Verification items for the finished model (mm, model axes). A direction names the side the tool comes from. Round coordinates to 2 decimals unless told otherwise and drop trailing zeros. Order: outer loops, then holes, each group sorted by start corner. A loop starts at its lowest first (then second) coordinate and runs counter-clockwise, first axis right, second up. Notation, with made-up numbers: M 46,32 L 56,32 A21 ccw 56,41 Z; hole C 1.25,-22.5 d8. An arc over 180 degrees is marked long. Answer as a JSON object with one key per item and string values. Group by question number.
```python
from build123d import *

# Parameters (mm, degrees)
F1_DEPTH = 38.1
F2_R     = 15.875
F3_DEPTH = 31.75
F5_DEPTH = 31.75


with BuildPart() as f1:
    # F0 (on Top) → F1 (new body)
    with BuildSketch(Plane.XY):
        with BuildLine():
            Line((17.5179102392, -5.2510727335), (17.5179102392, 5.2510727335))
            ThreePointArc((17.5179102392, 5.2510727335), (17.276294132, 5.9983835377), (17.0028141207, 6.7346310944))
            ThreePointArc((17.0028141207, 6.7346310944), (-18.288, 0), (17.0028141207, -6.7346310944))
            ThreePointArc((17.0028141207, -6.7346310944), (17.276294132, -5.9983835377), (17.5179102392, -5.2510727335))
        make_face()
        with BuildLine():
            ThreePointArc((17.0028141207, 6.7346310944), (17.276294132, 5.9983835377), (17.5179102392, 5.2510727335))
            ThreePointArc((17.5179102392, 5.2510727335), (23.5952406288, 0), (17.5179102392, -5.2510727335))
            ThreePointArc((17.5179102392, -5.2510727335), (17.276294132, -5.9983835377), (17.0028141207, -6.7346310944))
            ThreePointArc((17.0028141207, -6.7346310944), (25.1441620986, 0), (17.0028141207, 6.7346310944))
        make_face()
    extrude(amount=-F1_DEPTH)

    # F2 (on face) → F3 (cut)
    with BuildSketch(Plane(origin=(0, 0, -38.1), x_dir=(1, 0, 0), z_dir=(0, 0, -1))):
        Circle(F2_R)
    extrude(amount=-F3_DEPTH, mode=Mode.SUBTRACT)

    # F4 (on face) → F5 (cut)
    with BuildSketch(Plane(origin=(0, 0, -38.1), x_dir=(1, 0, 0), z_dir=(0, 0, -1))):
        with BuildLine():
            ThreePointArc((17.0028141207, -6.7346310944), (25.1441620986, 0), (17.0028141207, 6.7346310944))
            Line((17.0028141207, 6.7346310944), (17.5179102392, 5.2510727335))
            ThreePointArc((17.5179102392, 5.2510727335), (23.5952406288, 0), (17.5179102392, -5.2510727335))
            Line((17.5179102392, -5.2510727335), (17.0028141207, -6.7346310944))
        make_face()
    extrude(amount=-F5_DEPTH, mode=Mode.SUBTRACT)


solid = f1.part
```
Q1. Gauge pin test, flat ends, axial feed: pin 1 Ø12 at (y, z) = (-5, -28) entering from -X; pin 2 Ø1.5 at (y, z) = (7, -29.5) entering from -X; pin 3 Ø3 at (y, z) = (13, -25.5) entering from -X. Record the tip position at first contact, or that the pin passes through.
Q2. Cross-section at C-C, the plane z = -20. Record the cut outline in (x, y) (3 decimals), then the cut area to 3 significant figures.
Q3. Tool access check on faces 1 (the face through (17.257, -6.003, -22.447)), 2 (the face through (-15, 6, -38.1)), 3 (the face through (0, 0, -6.35)). Record the directions out of +Z, -Z, +X, -X, +Y, -Y that give a thin tool (end or side, any length) a straight path to the whole face; none if there is none.
Q4. Cross-section at D-D, the plane x = 21.5. Record the cut outline in (y, z).
Q5. Thickness scan on line 1 (X direction, y = 0, z = -23) (3 decimals); line 2 (Y direction, x = 0, z = -25) (3 decimals); line 3 (Z direction, x = 12.5, y = -3). Record the ranges inside material, lowest first. Write a range as from..to.
Q6. Cross-section at A-A, the plane y = 0. Record the cut outline in (x, z) (3 decimals).
Q7. Cross-section at B-B, the plane x = 0. Record the cut outline in (y, z) (3 decimals).
Q8. Release check for a two-part mould opening along X. For faces 4 (the face through (-2, 0, 0)), 5 (the face through (17.518, 0, -19)), 6 (the face through (17.264, 5.982, -22.447)), 7 (the face through (-3.441, 15.497, -22.447)) record: released by +X, released by -X, zero draft, split by the parting line, or undercut.
Conclusion:
{
 "1": {"pin 1": "x = -18.29", "pin 2": "x = -17.19", "pin 3": "x = -14.22"},
 "2": {"outline": "M 17.003,-6.735 L 17.518,-5.251 L 17.518,5.251 L 17.003,6.735 A18.288 ccw long Z; hole C 0,0 d31.75", "area": "254 mm2"},
 "3": {"face 1": "-Z, +X, -Y", "face 2": "-Z, +X, -X, +Y, -Y", "face 3": "-Z"},
 "4": {"outline": "M -6.06,-6.35 L -4.22,-6.35 L -4.22,0 L -6.06,0 Z; M 4.22,-6.35 L 6.06,-6.35 L 6.06,0 L 4.22,0 Z"},
 "5": {"line 1": "-18.288..-15.875, 15.875..17.518", "line 2": "-18.288..-15.875, 15.875..18.288", "line 3": "-6.35..0"},
 "6": {"outline": "M -18.288,-38.1 L -15.875,-38.1 L -15.875,-6.35 L 15.875,-6.35 L 15.875,-38.1 L 17.518,-38.1 L 17.518,0 L -18.288,0 Z; M 23.595,-6.35 L 25.144,-6.35 L 25.144,0 L 23.595,0 Z"},
 "7": {"outline": "M -18.288,-38.1 L -15.875,-38.1 L -15.875,-6.35 L 15.875,-6.35 L 15.875,-38.1 L 18.288,-38.1 L 18.288,0 L -18.288,0 Z"},
 "8": {"face 4": "zero draft", "face 5": "undercut", "face 6": "released by +X", "face 7": "undercut"}
}
